Geometry check sheet. Reference: the model listing, model coordinates, mm. A direction names the side the tool comes from. Round coordinates to 2 decimals unless told otherwise and drop trailing zeros. Write each loop counter-clockwise with the first axis right and the second up, starting at its lowest first coordinate (ties: lowest second). Pieces come first, ordered by that corner, then holes. Notation, with made-up numbers: M 49.5,72 L 62.5,72 A29 cw 62.5,108 Z; hole C 57,29 d5. An arc over 180 degrees is marked long. Put each result on its own line as item: value. Start each with the question number.
(1) Gauge pin test, flat ends, axial feed: pin 1 (1.3 mm diameter, centred on x = 10.5, z = 50.5, fed in from +Y); pin 2 (2 mm diameter, centred on y = -10, z = 42, fed in from -X); pin 3 (6 mm diameter, centred on y = -4.5, z = 7.5, fed in from +X). Record the tip position at first contact, or that the pin passes through.
(2) Tool access check on faces 1 (the flat face through (1.5, -10, 36)), 2 (the flat face through (-7, -7, 2)), 3 (the flat face through (7, 7, 2)). Record the directions out of +Z, -Z, +X, -X, +Y, -Y that give a thin tool (end or side, any length) a straight path to the whole face; none if there is none.
(3) Material ranges on probe 1 along Z at (x, y) = (7.5, 7.5); probe 2 along X at (y, z) = (4.5, 29.5); probe 3 along Y at (x, z) = (5.5, 54.5), recorded low to high.
(4) Section check A-A on y = 0. Record the cut outline in (x, z), then the cut area to 3 significant figures.
(5) Section check B-B on z = 9. Record the cut outline in (x, y).
from build123d import *

# Parameters (mm, degrees)
SKETCH023_R             = 11.75
SKETCH023_R_2           = 9.25
PAD015_DEPTH            = 70
SKETCH025_W             = 31.48
SKETCH025_H             = 3
POCKET007_DEPTH         = 67
CHAMFER006_SIZE         = 2
SKETCH024_W             = 13.153862
SKETCH024_H             = 12.44
POCKET006_DEPTH         = 67
BODY013_PLACEMENT_ANGLE = 180


with BuildPart() as part:
    # Sketch023 → Pad015 (new body)
    with BuildSketch(Plane.XY):
        Circle(SKETCH023_R)
        Circle(SKETCH023_R_2, mode=Mode.SUBTRACT)
    extrude(amount=PAD015_DEPTH)

    # Sketch025 (on Face3 of Pad015) → Pocket007 (cut)
    with BuildSketch(Plane(origin=(0, 0, 0), x_dir=(1, 0, 0), z_dir=(0, 0, -1))):
        Rectangle(SKETCH025_W, SKETCH025_H)
    extrude(amount=-POCKET007_DEPTH, mode=Mode.SUBTRACT)

    # Chamfer006
    chamfer006_edges = [part.edges().sort_by_distance(p)[0] for p in [
        (0, 11.75, 0),
        (0, -11.75, 0),
    ]]
    chamfer(chamfer006_edges, length=CHAMFER006_SIZE)

    # Sketch024 (on Face11 of Chamfer006) → Pocket006 (cut)
    with BuildSketch(Plane(origin=(0, 0, 0), x_dir=(1, 0, 0), z_dir=(0, 0, -1))):
        with Locations((5.076931, 7.72)):
            Rectangle(SKETCH024_W, SKETCH024_H)
        with Locations((-5.076931, -7.72)):
            Rectangle(SKETCH024_W, SKETCH024_H)
    extrude(amount=-POCKET006_DEPTH, mode=Mode.SUBTRACT)


with BuildPart() as part_1:
    # Body013 placement: moved
    add(part.part.moved(Location((0, 0, 69))).rotate(Axis((0, 0, 69), (1, 0, 0)), BODY013_PLACEMENT_ANGLE))


solid = part_1.part
Answers follow:
1. pin 1: stops at y = -1.5
1. pin 2: stops at x = 1.5
1. pin 3: stops at x = 11.65
2. face 1: +Z, -X, +Y, -Y
2. face 2: +Z, -X, -Y
2. face 3: +Z, +X, +Y
3. probe 1: z = -1 to 2
3. probe 2: x = -10.85 to -8.08
3. probe 3: y = -10.38 to -7.44
4. outline: M -11.75,-1 L -9.25,-1 L -9.25,2 L -11.75,2 Z; M 9.25,-1 L 11.75,-1 L 11.75,2 L 9.25,2 Z
4. area: 15.0 mm^2
5. outline: M -11.65,1.5 L -9.13,1.5 A9.25 cw -1.5,9.13 L -1.5,11.65 A11.75 ccw Z; M 1.5,-11.65 A11.75 ccw 11.65,-1.5 L 9.13,-1.5 A9.25 cw 1.5,-9.13 Z
